```python
from build123d import *

# Parameters (mm, degrees)
SKETCH4_W                = 12.46
SKETCH4_H                = 17.25
BOSS_EXTRUDE3_DEPTH      = 6
SKETCH8_R                = 12.546781182
SKETCH8_R_2              = 11.15
BOSS_EXTRUDE6_DEPTH      = 8.3
BOSS_EXTRUDE6_DEPTH_BACK = 17.25
BOSS_EXTRUDE4_DEPTH      = 17.25
SKETCH6_R                = 0.75
CUT_EXTRUDE1_DEPTH       = 5
CHAMFER1_SIZE            = 0.5
CHAMFER1_SIZE2           = 0.866025404
SKETCH10_W               = 12.46
SKETCH10_H               = 23.7
CUT_EXTRUDE3_DEPTH       = 17.25
BOSS_EXTRUDE7_DEPTH      = 8.3
BOSS_EXTRUDE9_DEPTH      = 10
SKETCH16_R               = 11.15
SKETCH16_R_2             = 7.2
BOSS_EXTRUDE10_DEPTH     = 8.3
SKETCH17_R               = 10.2
SKETCH17_R_2             = 7.2
CUT_EXTRUDE5_DEPTH       = 1.3
SKETCH11_W               = 10
SKETCH11_H               = 2
CUT_EXTRUDE4_DEPTH       = 23.7
CUT_EXTRUDE7_REACH       = 37.55
SKETCH19_W               = 12.46
SKETCH19_H               = 6
OFFSET_R_DEPTH           = 10
SKETCH21_R               = 30
SKETCH21_R_2             = 25
CUT_EXTRUDE9_DEPTH       = 5
SKETCH22_W               = 12
SKETCH22_H               = 6
CUT_EXTRUDE10_DEPTH      = 11
SKETCH20_R               = 10
CUT_EXTRUDE8_DEPTH       = 10
FILLET1_R                = 1
CUT_EXTRUDE11_DEPTH      = 11
SKETCH24_R               = 0.75
CUT_EXTRUDE12_DEPTH      = 11
SKETCH25_R               = 1.5
CUT_EXTRUDE13_DEPTH      = 7


with BuildPart() as part:
    # Sketch4 → Boss-Extrude3 (new body)
    with BuildSketch(Plane.XY):
        with Locations((0, -1.35)):
            Rectangle(SKETCH4_W, SKETCH4_H)
    extrude(amount=BOSS_EXTRUDE3_DEPTH)



with BuildPart() as body_2:
    # Sketch8 → Boss-Extrude6 (new body, two sides)
    with BuildSketch(Plane(origin=(0, -9.975, 0), x_dir=(-1, 0, 0), z_dir=(0, -1, 0))) as boss_extrude6_sk:
        with Locations((0, -23.55)):
            Circle(SKETCH8_R)
        with Locations((0, -23.55)):
            Circle(SKETCH8_R_2, mode=Mode.SUBTRACT)
    extrude(amount=BOSS_EXTRUDE6_DEPTH)
    extrude(boss_extrude6_sk.sketch, amount=-BOSS_EXTRUDE6_DEPTH_BACK)


with BuildPart() as part_1:
    add(part.part)

    add(body_2.part)  # Boss-Extrude4 merges body 2
    # Sketch5 → Boss-Extrude4 (add)
    with BuildSketch(Plane(origin=(0, 7.275, 0), x_dir=(1, 0, 0), z_dir=(0, 1, 0))):
        with BuildLine():
            Line((12.546781182, -23.55), (12.546781182, 0))
            Line((12.546781182, 0), (6.23, 0))
            Line((6.23, 0), (6.23, -29.7))
            Line((6.23, -29.7), (-6.23, -29.7))
            Line((-6.23, -29.7), (-6.23, 0))
            Line((-6.23, 0), (-12.546781182, 0))
            Line((-12.546781182, 0), (-12.546781182, -23.55))
            ThreePointArc((-12.546781182, -23.55), (0, -36.096781182), (12.546781182, -23.55))
        make_face()
    extrude(amount=-BOSS_EXTRUDE4_DEPTH)

    # Sketch6 → Cut-Extrude1 (cut)
    with BuildSketch(Plane(origin=(0, 7.275, 0), x_dir=(1, 0, 0), z_dir=(0, 1, 0))):
        with Locations((0, -3.6)):
            Circle(SKETCH6_R)
        with Locations((0, -32.1)):
            Circle(SKETCH6_R)
    extrude(amount=-CUT_EXTRUDE1_DEPTH, mode=Mode.SUBTRACT)

    # Chamfer1
    chamfer1_edges = [part_1.edges().sort_by_distance(p)[0] for p in [
        (-0.75, 7.275, 3.6),
        (-0.75, 7.275, 32.1),
    ]]
    chamfer1_side = [part_1.faces().sort_by_distance(p)[0] for p in [
        (0, 7.275, 35.657160381),
    ]]
    chamfer(chamfer1_edges, length=CHAMFER1_SIZE, length2=CHAMFER1_SIZE2, reference=chamfer1_side[0])

    # Sketch10 → Cut-Extrude3 (cut)
    with BuildSketch(Plane(origin=(0, 7.275, 0), x_dir=(1, 0, 0), z_dir=(0, 1, 0))):
        with Locations((0, -17.85)):
            Rectangle(SKETCH10_W, SKETCH10_H)
    extrude(amount=-CUT_EXTRUDE3_DEPTH, mode=Mode.SUBTRACT)

    # Sketch13 → Boss-Extrude7 (add)
    with BuildSketch(Plane.XZ.offset(18.275)):
        with BuildLine():
            Line((-12.546781182, 23.55), (-12.546781182, 0))
            Line((-12.546781182, 0), (12.546781182, 0))
            Line((12.546781182, 0), (12.546781182, 23.55))
            ThreePointArc((12.546781182, 23.55), (0, 11.003218818), (-12.546781182, 23.55))
        make_face()
    extrude(amount=-BOSS_EXTRUDE7_DEPTH)

    # Sketch15 → Boss-Extrude9 (add)
    with BuildSketch(Plane(origin=(0, 7.275, 0), x_dir=(1, 0, 0), z_dir=(0, 1, 0))):
        with BuildLine():
            Line((-12.546781182, 0), (12.546781182, 0))
            Line((12.546781182, 0), (12.546781182, -23.55))
            ThreePointArc((12.546781182, -23.55), (0, -36.096781182), (-12.546781182, -23.55))
            Line((-12.546781182, -23.55), (-12.546781182, 0))
        make_face()
        with BuildLine():
            Line((-6.23, -0.8), (6.23, -0.8))
            Line((6.23, -0.8), (6.23, -33))
            ThreePointArc((6.23, -33), (5.790660172, -34.060660172), (4.73, -34.5))
            Line((4.73, -34.5), (-4.73, -34.5))
            ThreePointArc((-4.73, -34.5), (-5.790660172, -34.060660172), (-6.23, -33))
            Line((-6.23, -33), (-6.23, -0.8))
        make_face(mode=Mode.SUBTRACT)
    extrude(amount=BOSS_EXTRUDE9_DEPTH)

    # Sketch16 → Boss-Extrude10 (add)
    with BuildSketch(Plane.XZ.offset(18.275)):
        with Locations((0, 23.55)):
            Circle(SKETCH16_R)
        with Locations((0, 23.55)):
            Circle(SKETCH16_R_2, mode=Mode.SUBTRACT)
    extrude(amount=-BOSS_EXTRUDE10_DEPTH)

    # Sketch17 → Cut-Extrude5 (cut)
    with BuildSketch(Plane.XZ.offset(18.275)):
        with Locations((0, 23.55)):
            Circle(SKETCH17_R)
        with Locations((0, 23.55)):
            Circle(SKETCH17_R_2, mode=Mode.SUBTRACT)
    extrude(amount=-CUT_EXTRUDE5_DEPTH, mode=Mode.SUBTRACT)

    # Sketch11 → Cut-Extrude4 (cut)
    with BuildSketch(Plane.XY.offset(29.7)):
        with Locations((0, -10.975)):
            Rectangle(SKETCH11_W, SKETCH11_H)
    extrude(amount=-CUT_EXTRUDE4_DEPTH, mode=Mode.SUBTRACT)

    # Sketch19 → Cut-Extrude7 (cut, up to next)
    with BuildSketch(Plane.XZ.offset(18.275), mode=Mode.PRIVATE) as cut_extrude7_sk1:
        with Locations((0, 9)):
            Rectangle(SKETCH19_W, SKETCH19_H)
    cut_extrude7_tool1 = extrude(cut_extrude7_sk1.sketch, amount=-CUT_EXTRUDE7_REACH, mode=Mode.PRIVATE) & part_1.part
    add(cut_extrude7_tool1.solids().sort_by_distance((0, -18.275, 9))[0], mode=Mode.SUBTRACT)

    # Sketch1 → Offset R (add)
    with BuildSketch(Plane.XY):
        Polygon((0, -75), (70.674424412, 22.275), (-70.674424412, 22.275), align=None)
    extrude(amount=-OFFSET_R_DEPTH)

    # Sketch21 → Cut-Extrude9 (cut)
    with BuildSketch(Plane.XY):
        with Locations((0, -75)):
            Circle(SKETCH21_R)
        with Locations((0, -75)):
            Circle(SKETCH21_R_2, mode=Mode.SUBTRACT)
    extrude(amount=-CUT_EXTRUDE9_DEPTH, mode=Mode.SUBTRACT)

    # Sketch22 → Cut-Extrude10 (cut, through all)
    with BuildSketch(Plane.XY):
        with Locations((0, -26.275)):
            Rectangle(SKETCH22_W, SKETCH22_H)
    extrude(amount=-CUT_EXTRUDE10_DEPTH, mode=Mode.SUBTRACT)

    # Sketch20 → Cut-Extrude8 (cut)
    with BuildSketch(Plane.XY):
        with Locations((0, -75)):
            Circle(SKETCH20_R)
    extrude(amount=-CUT_EXTRUDE8_DEPTH, mode=Mode.SUBTRACT)

    # Fillet1
    fillet1_edges = [part_1.edges().sort_by_distance(p)[0] for p in [
        (5.877852523, -66.909830056, -5),
        (-5.877852523, -66.909830056, -5),
    ]]
    fillet(fillet1_edges, radius=FILLET1_R)

    # Sketch23 → Cut-Extrude11 (cut, through all)
    with BuildSketch(Plane.XY):
        Polygon((-35.407309274, 22.275), (-53.040866843, -1.995509831), (-70.674424412, 22.275), align=None)
        Polygon((70.674424412, 22.275), (35.407309274, 22.275), (53.040866843, -1.995509831), align=None)
    extrude(amount=-CUT_EXTRUDE11_DEPTH, mode=Mode.SUBTRACT)

    # Sketch24 → Cut-Extrude12 (cut, through all)
    with BuildSketch(Plane.XY):
        with Locations((-28.040866843, -1.995509831)):
            Circle(SKETCH24_R)
        with Locations((28.040866843, -1.995509831)):
            Circle(SKETCH24_R)
    extrude(amount=-CUT_EXTRUDE12_DEPTH, mode=Mode.SUBTRACT)

    # Sketch25 → Cut-Extrude13 (cut)
    with BuildSketch(Plane.XY):
        with Locations((-28.040866843, -1.995509831)):
            Circle(SKETCH25_R)
        with Locations((28.040866843, -1.995509831)):
            Circle(SKETCH25_R)
    extrude(amount=-CUT_EXTRUDE13_DEPTH, mode=Mode.SUBTRACT)


solid = part_1.part
```
Here's how the part is built. I have some questions about the finished solid (model axes, mm). A direction names the side the tool comes from. Round coordinates to 2 decimals unless told otherwise and drop trailing zeros. Loops run counter-clockwise (first coordinate to the right, second up) from the corner with the lowest first, then second, coordinate; pieces in that order, holes last. Notation, with made-up numbers: (84, 69) -> (132, 69) arc R22 cw to (132, 103) -> close; hole circle Ø7 at (48, 27). An arc over 180 degrees is marked (long way). Answer as CSV lines item,"result". Start each with the question number.
1. I need wall thicknesses on probe 1 along Z at (x, y) = (0, 4); probe 2 along Z at (x, y) = (25.5, 0); probe 3 along X at (y, z) = (0.5, 11). Which ranges of each line are inside material? Lowest first, please. Write a range as from..to.
2. Imagine slicing it at C-C on y = 4.5. Write out the boundary of the cut face in (x, z).
3. I'm going to push flat-ended pins straight in: P1, Ø18, axis at x = -3, y = -57.5, coming from the +Z side; P2, Ø1, axis at x = -10, y = -5.5, coming from the +Z side; P3, Ø1, axis at y = -11.5, z = 16.5, coming from the +X side. Where does each tip first touch, or does it pass through?
4. For faces 1 (the face through (-12.547, -1, 12)), 2 (the face through (0, -23.275, -5)), 3 (the face through (0, -15, 12)), 4 (the face through (0, -2, 29.7)), 5 (the face through (0, -45, -2)), which set-ups out of +Z, -Z, +X, -X, +Y, -Y let a thin tool reach every point of the face, with its end or its side?
5. Imagine slicing it at D-D on x = 43. Write out the boundary of the cut face in (y, z).
6. If we mould it in two halves opening along Y, with no side actions, what happens to faces 6 (the face through (0, 12, 0.8)), 7 (the face through (29.41, -34.52, -4.93)), 8 (the face through (0, -29.275, -5)), 9 (the face through (0, 7.275, 2))? For each: pulls with the +Y half, pulls with the -Y half, needs draft (parallel to the pull), parting line crosses it, or undercut.
7. Imagine slicing it at B-B on y = -5.5. Write out the boundary of the cut face in (x, z), plus the area to 3 significant figures.
8. Imagine slicing it at A-A on z = -2. Write out the boundary of the cut face in (x, y) (1 decimal), plus the area to 3 significant figures.
Solution:
1,probe 1,"-10..2.85, 4.35..6, 29.7..31.35, 32.85..36.1"
1,probe 2,"-10..0"
1,probe 3,"-12.55..-6.23, 6.23..12.55"
2,outline,"(-48.32, -10) -> (48.32, -10) -> (48.32, 0) -> (12.55, 0) -> (12.55, 23.55) arc R12.55 ccw to (-12.55, 23.55) -> (-12.55, 0) -> (-48.32, 0) -> close; hole (-6.23, 6) -> (6.23, 6) -> (6.23, 29.7) -> (-6.23, 29.7) -> close; hole circle Ø1.5 at (0, 3.6); hole circle Ø1.5 at (0, 32.1)"
3,P1,"z = 0"
3,P2,"z = 31.75"
3,P3,"x = 12.55"
4,face 1,"+Z, -X, +Y, -Y"
4,face 2,"+Z, -Z"
4,face 3,"+Y, -Y"
4,face 4,"+Y"
4,face 5,"+Z"
5,outline,"(-15.82, -10) -> (11.82, -10) -> (11.82, 0) -> (-15.82, 0) -> close"
6,face 6,"needs draft"
6,face 7,"pulls with the -Y half"
6,face 8,"undercut"
6,face 9,"pulls with the +Y half"
7,outline,"(-50.49, -10) -> (50.49, -10) -> (50.49, 0) -> (12.55, 0) -> (12.55, 23.55) arc R12.55 ccw to (-12.55, 23.55) -> (-12.55, 0) -> (-50.49, 0) -> close; hole (-6.23, 6) -> (6.23, 6) -> (6.23, 29.7) -> (-6.23, 29.7) -> close"
7,area,"1,550 mm²"
8,outline,"(-53, -2) -> (-17.6, -50.7) arc R30 cw to (17.6, -50.7) -> (53, -2) -> (35.4, 22.3) -> (-35.4, 22.3) -> close; (-14.7, -54.8) -> (-6.4, -66.1) arc R1 ccw to (-5.1, -66.4) arc R10 cw to (5.1, -66.4) arc R1 ccw to (6.4, -66.1) -> (14.7, -54.8) arc R25 ccw to start; hole circle Ø3 at (-28, -2); hole (-6, -29.3) -> (6, -29.3) -> (6, -23.3) -> (-6, -23.3) -> close; hole circle Ø3 at (28, -2)"
8,area,"5,700 mm²"
